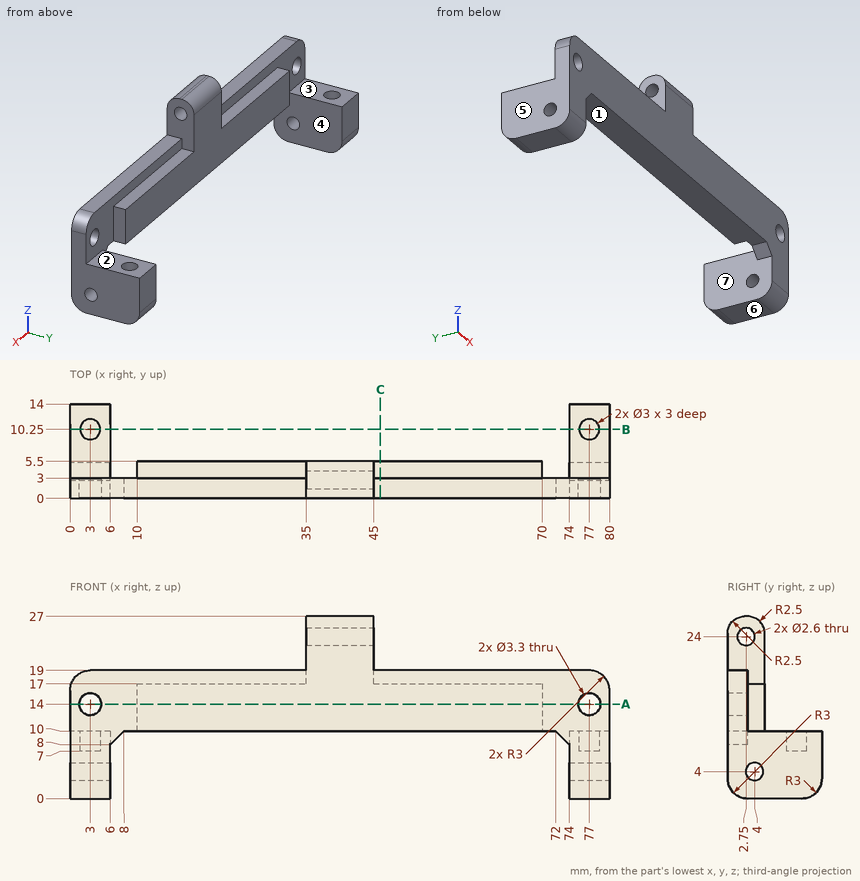
For this review, use the dimensioned drawing (mm, ordinates from the lowest corner) and the shaded views. A direction names the side the tool comes from. Coordinates: 2 decimals unless noted, no trailing zeros. Order: outer loops, then holes, each group sorted by start corner. A loop starts at its lowest first (then second) coordinate and runs counter-clockwise, first axis right, second up. Notation, with made-up numbers: (69.5, 22.25) -> (83.5, 22.25) arc R19 ccw to (83.5, 40.25) -> close; hole circle Ø11 at (-16, -17.5). An arc over 180 degrees is marked (long way). One line per item, written item: value. Start each with the question number.
Q1. Tool access review of the marked faces 1, 2, 3 and 4: name each direction out of +Z, -Z, +X, -X, +Y, -Y from which nothing blocks a thin tool from reaching the whole face with its end or side.
Q2. Take a section at A-A, the plane z = 14. State the section outline as (x, y) points.
Q3. Take a section at B-B, the plane y = 10.25. State the section outline as (x, z) points.
Q4. For probe 1 along X at (y, z) = (6.25, 7.5); probe 2 along Z at (x, y) = (78.7, 4); probe 3 along X at (y, z) = (4, 21.75), list the stretches that pass through material, from the lowest coordinate up.
Q5. Take a section at C-C, the plane x = 46. State the section outline as (y, z) points.
Q6. Insertion check: pin 1 Ø5 at (x, y) = (4, 8) entering from +Z; pin 2 Ø1.6 at (x, y) = (50.5, 2.5) entering from -Z; pin 3 Ø1.2 at (y, z) = (5, 12.5) entering from -X. Each pin has a flat end and moves straight along its axis. Give the tip position at first contact, or say it passes through.
Q7. Mouldability with a two-part tool opening along X and no side actions: class the marked faces 5, 6 and 7 as pulls with the +X half, pulls with the -X half, needs draft (parallel to the pull), parting line crosses it, or undercut.
Values follow:
1. face 1: -Z, +Y, -Y
1. face 2: +Z, +X, +Y
1. face 3: +Z, -X, +Y
1. face 4: -Z, +Y
2. outline: (0, 0) -> (1.35, 0) -> (1.35, 3) -> (0, 3) -> close; (4.65, 0) -> (75.35, 0) -> (75.35, 3) -> (70, 3) -> (70, 5.5) -> (10, 5.5) -> (10, 3) -> (4.65, 3) -> close; (78.65, 0) -> (80, 0) -> (80, 3) -> (78.65, 3) -> close
3. outline: (0, 0) -> (6, 0) -> (6, 10) -> (4.5, 10) -> (4.5, 7) -> (1.5, 7) -> (1.5, 10) -> (0, 10) -> close; (74, 0) -> (80, 0) -> (80, 10) -> (78.5, 10) -> (78.5, 7) -> (75.5, 7) -> (75.5, 10) -> (74, 10) -> close
4. probe 1: x = 0 to 6, 74 to 80
4. probe 2: z = 0 to 2.7, 5.3 to 10
4. probe 3: x = 35 to 45
5. outline: (0, 10) -> (5.5, 10) -> (5.5, 17) -> (3, 17) -> (3, 19) -> (0, 19) -> close
6. pin 1: stops at z = 10
6. pin 2: stops at z = 10
6. pin 3: stops at x = 10
7. face 5: pulls with the -X half
7. face 6: needs draft
7. face 7: undercut
